Here's the drawing with two shaded views (mm, measured from the low corner). I have some questions. A direction names the side the tool comes from. Round coordinates to 2 decimals unless told otherwise and drop trailing zeros. Loops run counter-clockwise (first coordinate to the right, second up) from the corner with the lowest first, then second, coordinate; pieces in that order, holes last.
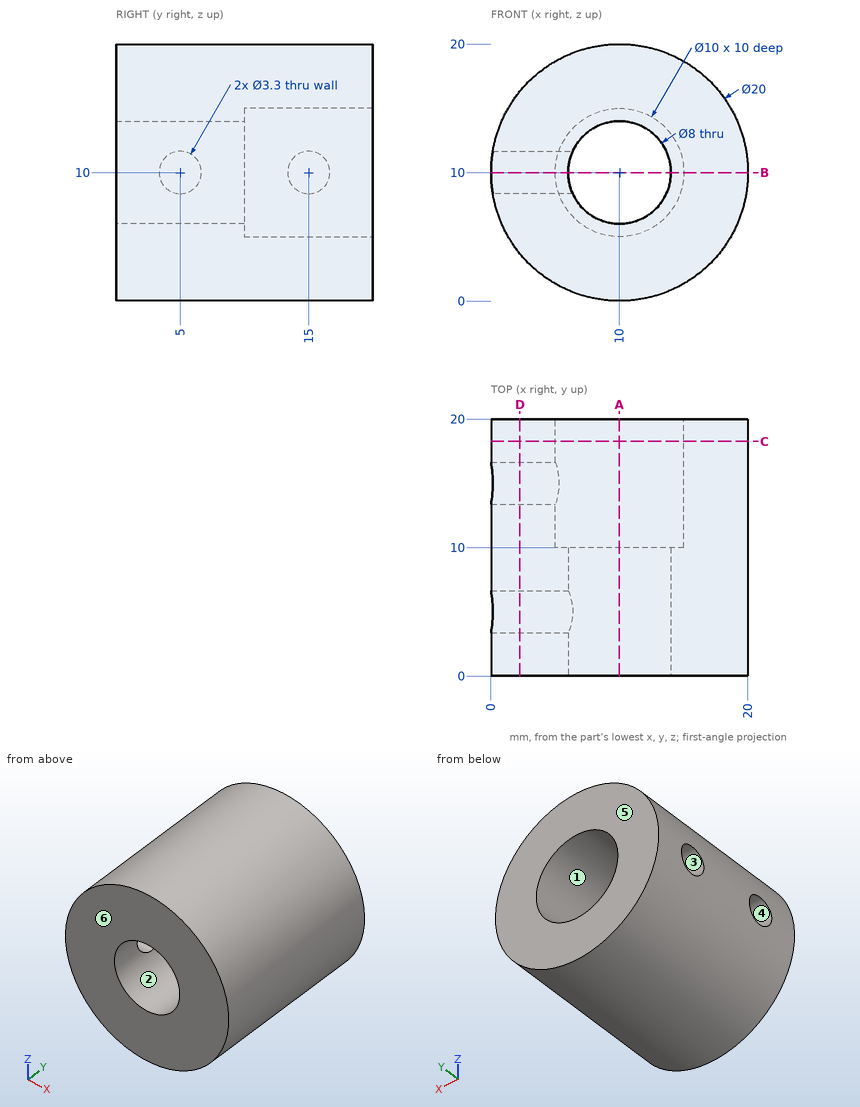
(1) Will these pins go through, and if not, where does the flat tip stop? P1, Ø8, axis at x = 4, y = 6, coming from the -Z side; P2, Ø9, axis at x = 10, z = 10, coming from the +Y side; P3, Ø6, axis at y = 9.5, z = 7, coming from the -X side; P4, Ø1.5, axis at x = 15.5, y = 5.5, coming from the -Z side.
Worked answers:
P1: stops at z = 0.2
P2: stops at y = 10
P3: stops at x = 0
P4: stops at z = 1.2
(2) If we section it at A-A, the plane x = 10: List the corners of the cut face in (y, z) for me, then the cut area to 3 significant figures.
Worked answers:
outline: (0, 0) - (20, 0) - (20, 5) - (10, 5) - (10, 6) - (0, 6) - close; (0, 14) - (10, 14) - (10, 15) - (20, 15) - (20, 20) - (0, 20) - close
area: 220 mm2
(3) If we section it at D-D, the plane x = 2.25: List the corners of the cut face in (y, z) for me.
Worked answers:
outline: (0, 3.68) - (20, 3.68) - (20, 16.32) - (0, 16.32) - close; hole circle Ø3.3 at (5, 10); hole circle Ø3.3 at (15, 10)
(4) If we section it at B-B, the plane z = 10: List the corners of the cut face in (x, y) for me.
Worked answers:
outline: (0, 0) - (6, 0) - (6, 3.35) - (0, 3.35) - close; (0, 6.65) - (6, 6.65) - (6, 10) - (5, 10) - (5, 13.35) - (0, 13.35) - close; (0, 16.65) - (5, 16.65) - (5, 20) - (0, 20) - close; (14, 0) - (20, 0) - (20, 20) - (15, 20) - (15, 10) - (14, 10) - close
(5) If we mould it in two halves opening along Y, with no side actions, what happens to the marked faces 3, 4, 5 and 6? For each: released by +Y, released by -Y, zero draft, split by the parting line, or undercut.
Worked answers:
face 3: undercut
face 4: undercut
face 5: released by +Y
face 6: released by -Y
(6) If we section it at C-C, the plane y = 18.25: List the corners of the cut face in (x, z) for me, then the cut area to 3 significant figures.
Worked answers:
outline: circle Ø20 at (10, 10); hole circle Ø10 at (10, 10)
area: 236 mm2
(7) If I drill on line 1 (Y direction, x = 4.1, z = 10); line 2 (X direction, y = 16, z = 10); line 3 (Z direction, x = 2, y = 3.5), over which ranges is the centre line in solid material (lowest first)?
Worked answers:
line 1: y = 0 to 3.35, 6.65 to 13.35, 16.65 to 20
line 2: x = 15 to 20
line 3: z = 4 to 9.31, 10.69 to 16
(8) For the marked faces 1 and 2, which set-ups out of +Z, -Z, +X, -X, +Y, -Y let a thin tool reach every point of the face, with its end or its side?
Worked answers:
face 1: +Y
face 2: +Y, -Y
